from build123d import *

# Parameters (mm, degrees)
BOSS_EXTRUDE1_DEPTH = 100
FILLET1_R           = 1


with BuildPart() as part:
    # Sketch1 → Boss-Extrude1 (new body)
    with BuildSketch(Plane.XY.offset(115.120373728)):
        with BuildLine():
            Line((43.606003854, 44.364343494), (40.289379064, 44.364343494))
            ThreePointArc((40.289379064, 44.364343494), (41.947691459, 38.864343494), (43.606003854, 44.364343494))
        make_face()
    extrude(amount=-BOSS_EXTRUDE1_DEPTH)

    # Fillet1
    # the kernel refuses this fillet: 1 mm, written as the material it takes off along each edge
    with BuildSketch(Plane(origin=(46.106003854, 44.364343494, 115.120373728), x_dir=(0, 0, -1), z_dir=(-1, 0, 0))) as fillet1_piece_1:
        with BuildLine():
            CenterArc((FILLET1_R, FILLET1_R), FILLET1_R, 180, 90)
            Line((0, FILLET1_R), (0, 0))
            Line((0, 0), (FILLET1_R, 0))
        make_face()
    extrude(amount=8.31662479, mode=Mode.SUBTRACT)
    with BuildSketch(Plane(origin=(41.947691459, 41.864343494, 115.120373728), x_dir=(-0.0031415874858803736, 0.9999950652018582, 0), z_dir=(0.9999950652018582, 0.0031415874858803736, 0))) as fillet1_piece_2:
        with BuildLine():
            CenterArc((3 - FILLET1_R, -FILLET1_R), FILLET1_R, 0, 90)
            Line((3 - FILLET1_R, 0), (3, 0))
            Line((3, 0), (3, -FILLET1_R))
        make_face()
    revolve(axis=Axis((41.947691459, 41.864343494, 115.120373728), (0, 0, 1)), revolution_arc=359.64, mode=Mode.SUBTRACT)
    with BuildSketch(Plane(origin=(41.947691459, 41.864343494, 15.120373728), x_dir=(-0.0031415874858803736, 0.9999950652018582, 0), z_dir=(0.9999950652018582, 0.0031415874858803736, 0))) as fillet1_piece_3:
        with BuildLine():
            CenterArc((3 - FILLET1_R, FILLET1_R), FILLET1_R, 270, 90)
            Line((3 - FILLET1_R, 0), (3, 0))
            Line((3, 0), (3, FILLET1_R))
        make_face()
    revolve(axis=Axis((41.947691459, 41.864343494, 15.120373728), (0, 0, 1)), revolution_arc=359.64, mode=Mode.SUBTRACT)
    with BuildSketch(Plane(origin=(46.106003854, 44.364343494, 15.120373728), x_dir=(0, 0, 1), z_dir=(-1, 0, 0))) as fillet1_piece_4:
        with BuildLine():
            CenterArc((FILLET1_R, -FILLET1_R), FILLET1_R, 90, 90)
            Line((0, -FILLET1_R), (0, 0))
            Line((0, 0), (FILLET1_R, 0))
        make_face()
    extrude(amount=8.31662479, mode=Mode.SUBTRACT)


solid = part.part
Model file for the job. Use its own axes, mm. Round coordinates to 2 decimals unless told otherwise and drop trailing zeros. Loops run counter-clockwise (first coordinate to the right, second up) from the corner with the lowest first, then second, coordinate; pieces in that order, holes last. Notation, with made-up numbers: (10.5, 28.25) -> (54.5, 28.25) arc R17 ccw to (54.5, 36.25) -> close; hole circle Ø11 at (22, -12). An arc over 180 degrees is marked (long way). Answer as CSV lines item,"result". Start each with the question number.
1) Probe line 1 along X through (y, z) = (44.1, 66.5); line 2 along X through (y, z) = (41.6, 38); line 3 along Z through (x, y) = (40.75, 44.05). List the from-to ranges inside material, lowest first.
2) Pin check, flat tip, straight feed: P1, Ø1, axis at y = 40.5, z = 52, coming from the +X side. Stop position of the tip, or through.
3) Slice it at A-A (z = 79). List the corners of the cut face in (x, y), plus the area to 3 significant figures.
Filled in:
1,line 1,"x = 39.95 to 43.95"
1,line 2,"x = 38.96 to 44.94"
1,line 3,"z = 15.39 to 114.85"
2,P1,"stops at x = 44.82"
3,outline,"(40.29, 44.36) arc R3 ccw (long way) to (43.61, 44.36) -> close"
3,area,"27.1 mm2"
